```python
from build123d import *

# Parameters (mm, degrees)
ESQUISSE1_W             = 17
ESQUISSE1_H             = 59
BOSS_EXTRU_1_DEPTH      = 2
ESQUISSE2_W             = 8.5
ESQUISSE2_H             = 59
BOSS_EXTRU_2_DEPTH      = 6
ESQUISSE3_W             = 1.5
ESQUISSE3_H             = 19.5
ESQUISSE3_H_2           = 11.5
ENL_V_MAT_EXTRU_1_DEPTH = 6
ESQUISSE4_R             = 2.25
ENL_V_MAT_EXTRU_2_DEPTH = 14
ENL_V_MAT_EXTRU_3_DEPTH = 6


with BuildPart() as part:
    # Esquisse1 → Boss.-Extru.1 (new body)
    with BuildSketch(Plane.XY):
        with Locations((8.5, -29.5)):
            Rectangle(ESQUISSE1_W, ESQUISSE1_H)
    extrude(amount=BOSS_EXTRU_1_DEPTH)

    # Esquisse2 → Boss.-Extru.2 (add)
    with BuildSketch(Plane.XY.offset(2)):
        with Locations((4.25, -29.5)):
            Rectangle(ESQUISSE2_W, ESQUISSE2_H)
    extrude(amount=BOSS_EXTRU_2_DEPTH)

    # Esquisse3 → Enlèv. mat.-Extru.1 (cut)
    with BuildSketch(Plane.XY.offset(8)):
        with Locations((2.75, -49.25)):
            Rectangle(ESQUISSE3_W, ESQUISSE3_H)
        with BuildLine():
            ThreePointArc((3.5, -37.202199257), (2.408191843, -38.127967907), (2, -39.5))
            Line((2, -39.5), (3.5, -39.5))
            Line((3.5, -39.5), (3.5, -37.202199257))
        make_face()
        with BuildLine():
            Line((3.5, -37.202199257), (3.5, -39.5))
            ThreePointArc((3.5, -39.5), (4.509962751, -38.490037249), (5.519925502, -39.5))
            Line((5.519925502, -39.5), (5.519925502, -37.202199257))
            ThreePointArc((5.519925502, -37.202199257), (4.509962751, -36.990037249), (3.5, -37.202199257))
        make_face()
        with BuildLine():
            Line((5.519925502, -37.202199257), (5.519925502, -39.5))
            Line((5.519925502, -39.5), (7.019925502, -39.5))
            ThreePointArc((7.019925502, -39.5), (6.611733659, -38.127967907), (5.519925502, -37.202199257))
        make_face()
        with Locations((6.269925502, -45.25)):
            Rectangle(ESQUISSE3_W, ESQUISSE3_H_2)
        with Locations((6.269925502, -13.75)):
            Rectangle(ESQUISSE3_W, ESQUISSE3_H_2)
        with Locations((2.75, -9.75)):
            Rectangle(ESQUISSE3_W, ESQUISSE3_H)
        with BuildLine():
            Line((3.5, -19.5), (2, -19.5))
            ThreePointArc((2, -19.5), (2.408191843, -20.872032093), (3.5, -21.797800743))
            Line((3.5, -21.797800743), (3.5, -19.5))
        make_face()
        with BuildLine():
            ThreePointArc((5.519925502, -19.5), (4.509962751, -20.509962751), (3.5, -19.5))
            Line((3.5, -19.5), (3.5, -21.797800743))
            ThreePointArc((3.5, -21.797800743), (4.509962751, -22.009962751), (5.519925502, -21.797800743))
            Line((5.519925502, -21.797800743), (5.519925502, -19.5))
        make_face()
        with BuildLine():
            Line((7.019925502, -19.5), (5.519925502, -19.5))
            Line((5.519925502, -19.5), (5.519925502, -21.797800743))
            ThreePointArc((5.519925502, -21.797800743), (6.611733659, -20.872032093), (7.019925502, -19.5))
        make_face()
    extrude(amount=-ENL_V_MAT_EXTRU_1_DEPTH, mode=Mode.SUBTRACT)

    # Esquisse4 → Enlèv. mat.-Extru.2 (cut)
    with BuildSketch(Plane.XY.offset(8)):
        with Locations((8.5, -33.5)):
            Circle(ESQUISSE4_R)
        with Locations((8.5, -25.5)):
            Circle(ESQUISSE4_R)
    extrude(amount=-ENL_V_MAT_EXTRU_2_DEPTH, mode=Mode.SUBTRACT)

    # Esquisse5 → Enlèv. mat.-Extru.3 (cut)
    with BuildSketch(Plane.XY.offset(8)):
        with BuildLine():
            Line((4.75, -25.5), (4.75, -33.5))
            ThreePointArc((4.75, -33.5), (5.848349571, -30.848349571), (8.5, -29.75))
            Line((8.5, -29.75), (8.5, -29.25))
            ThreePointArc((8.5, -29.25), (5.848349571, -28.151650429), (4.75, -25.5))
        make_face()
        with BuildLine():
            ThreePointArc((8.5, -21.75), (5.848349571, -22.848349571), (4.75, -25.5))
            ThreePointArc((4.75, -25.5), (5.848349571, -28.151650429), (8.5, -29.25))
            Line((8.5, -29.25), (8.5, -27.75))
            ThreePointArc((8.5, -27.75), (6.25, -25.5), (8.5, -23.25))
            Line((8.5, -23.25), (8.5, -21.75))
        make_face()
        with BuildLine():
            ThreePointArc((12.25, -25.5), (11.151650429, -22.848349571), (8.5, -21.75))
            Line((8.5, -21.75), (8.5, -23.25))
            ThreePointArc((8.5, -23.25), (6.25, -25.5), (8.5, -27.75))
            Line((8.5, -27.75), (8.5, -29.25))
            ThreePointArc((8.5, -29.25), (11.151650429, -28.151650429), (12.25, -25.5))
        make_face()
        with BuildLine():
            ThreePointArc((8.5, -29.75), (5.848349571, -30.848349571), (4.75, -33.5))
            ThreePointArc((4.75, -33.5), (5.848349571, -36.151650429), (8.5, -37.25))
            Line((8.5, -37.25), (8.5, -35.75))
            ThreePointArc((8.5, -35.75), (6.25, -33.5), (8.5, -31.25))
            Line((8.5, -31.25), (8.5, -29.75))
        make_face()
        with BuildLine():
            ThreePointArc((12.25, -33.5), (11.151650429, -30.848349571), (8.5, -29.75))
            Line((8.5, -29.75), (8.5, -31.25))
            ThreePointArc((8.5, -31.25), (6.25, -33.5), (8.5, -35.75))
            Line((8.5, -35.75), (8.5, -37.25))
            ThreePointArc((8.5, -37.25), (11.151650429, -36.151650429), (12.25, -33.5))
        make_face()
    extrude(amount=-ENL_V_MAT_EXTRU_3_DEPTH, mode=Mode.SUBTRACT)


solid = part.part
```
Check sheet for the modelled part. Datum: model origin and axes. Units: mm. A direction names the side the tool comes from. Coordinates: 2 decimals unless noted, no trailing zeros. Write each loop counter-clockwise with the first axis right and the second up, starting at its lowest first coordinate (ties: lowest second). Pieces come first, ordered by that corner, then holes. Notation, with made-up numbers: (6, 23.5) -> (54, 23.5) arc R17 cw to (54, 37.5) -> close; hole circle Ø11 at (33, 2). An arc over 180 degrees is marked (long way). Use a Markdown table: item, result.
1. Sectioned sample at A-A (y = -14). Enter the section's corners in (x, z).
Reported:
| item | result |
|---|---|
| outline | (0, 0) -> (17, 0) -> (17, 2) -> (8.5, 2) -> (8.5, 8) -> (7.02, 8) -> (7.02, 2) -> (5.52, 2) -> (5.52, 8) -> (3.5, 8) -> (3.5, 2) -> (2, 2) -> (2, 8) -> (0, 8) -> close |
2. Tool access check on faces 1 (the flat face through (8.5, -11, 5)), 2 (the flat face through (4.75, -29, 5)), 3 (the flat face through (3.5, -49, 5)), 4 (the flat face through (3.5, -10, 5)), 5 (the flat face through (7.02, -45, 5)). Record the directions out of +Z, -Z, +X, -X, +Y, -Y that give a thin tool (end or side, any length) a straight path to the whole face; none if there is none.
Reported:
| item | result |
|---|---|
| face 1 | +Z, +X, +Y, -Y |
| face 2 | +Z, +X |
| face 3 | +Z, -Y |
| face 4 | +Z, +Y |
| face 5 | +Z |
3. Scan lines: line 1 along Y through (x, z) = (8.5, 0.7); line 2 along X through (y, z) = (-15, 7.75); line 3 along Y through (x, z) = (7, 0.5). Record each from-to range of solid material in increasing order.
Reported:
| item | result |
|---|---|
| line 1 | y = -59 to -35.75, -31.25 to -27.75, -23.25 to 0 |
| line 2 | x = 0 to 2, 3.5 to 5.52, 7.02 to 8.5 |
| line 3 | y = -59 to -35.18, -31.82 to -27.18, -23.82 to 0 |
4. Sectioned sample at C-C (x = 10.25). Enter the section's corners in (y, z).
Reported:
| item | result |
|---|---|
| outline | (-59, 0) -> (-34.91, 0) -> (-34.91, 2) -> (-59, 2) -> close; (-32.09, 0) -> (-26.91, 0) -> (-26.91, 2) -> (-32.09, 2) -> close; (-24.09, 0) -> (0, 0) -> (0, 2) -> (-24.09, 2) -> close |
5. Go/stop test with flat-tipped pins: pin 1 Ø4 at (x, y) = (14, -31) entering from +Z; pin 2 Ø1.8 at (y, z) = (-14.5, 4) entering from +X; pin 3 Ø3.5 at (x, y) = (8.5, -25.5) entering from +Z. Record where each tip stops, or that it passes through.
Reported:
| item | result |
|---|---|
| pin 1 | stops at z = 2 |
| pin 2 | stops at x = 8.5 |
| pin 3 | passes through |
6. Release check for a two-part mould opening along Y. For faces 6 (the flat face through (2, -10, 5)), 7 (the cylindrical face through (5.9, -22.8, 5)), 8 (the flat face through (6, -59, 3)) record: pulls with the +Y half, pulls with the -Y half, needs draft (parallel to the pull), parting line crosses it, or undercut.
Reported:
| item | result |
|---|---|
| face 6 | needs draft |
| face 7 | undercut |
| face 8 | pulls with the -Y half |
7. Sectioned sample at B-B (z = 6.5). Enter the section's corners in (x, y), plus the area to 3 significant figures.
Reported:
| item | result |
|---|---|
| outline | (0, -59) -> (2, -59) -> (2, -39.5) arc R2.51 cw to (7.02, -39.5) -> (7.02, -51) -> (5.52, -51) -> (5.52, -39.5) arc R1.01 ccw to (3.5, -39.5) -> (3.5, -59) -> (8.5, -59) -> (8.5, -37.25) arc R3.75 cw to (4.75, -33.5) -> (4.75, -25.5) arc R3.75 cw to (8.5, -21.75) -> (8.5, 0) -> (3.5, 0) -> (3.5, -19.5) arc R1.01 ccw to (5.52, -19.5) -> (5.52, -8) -> (7.02, -8) -> (7.02, -19.5) arc R2.51 cw to (2, -19.5) -> (2, 0) -> (0, 0) -> close |
| area | 340 mm2 |
8. Sectioned sample at D-D (z = 0.5). Enter the section's corners in (x, y).
Reported:
| item | result |
|---|---|
| outline | (0, -59) -> (17, -59) -> (17, 0) -> (0, 0) -> close; hole circle Ø4.5 at (8.5, -33.5); hole circle Ø4.5 at (8.5, -25.5) |
